Verification items for the finished model (mm, model axes). A direction names the side the tool comes from. Round coordinates to 2 decimals unless told otherwise and drop trailing zeros. Order: outer loops, then holes, each group sorted by start corner. A loop starts at its lowest first (then second) coordinate and runs counter-clockwise, first axis right, second up. Notation, with made-up numbers: (-18.75, 2) -> (35.25, 2) arc R12 cw to (35.25, 23) -> close; hole circle Ø9 at (75.5, 55.5). An arc over 180 degrees is marked (long way). Put each result on its own line as item: value.
```python
from build123d import *

# Parameters (mm, degrees)
BOX_W     = 40
BOX_H     = 40
BOX_DEPTH = 3


with BuildPart() as cono:
    # Cone001 → Cone001 (revolve)
    with BuildSketch(Plane(origin=(0, 0, -4), x_dir=(1, 0, 0), z_dir=(0, -1, 0))):
        Polygon((0, 0), (16, 0), (3, 44), (0, 44), align=None)
    revolve(axis=Axis((0, 0, -4), (0, 0, 1)))


with BuildPart() as cone:
    # Cone → Cone (revolve)
    with BuildSketch(Plane.XZ):
        Polygon((0, 0), (16, 0), (4, 40), (0, 40), align=None)
    revolve(axis=Axis((0, 0, 0), (0, 0, 1)))


with BuildPart() as cut:
    # Box → Box (new body)
    with BuildSketch(Plane(origin=(-20, -20, 0), x_dir=(1, 0, 0), z_dir=(0, 0, 1))):
        with Locations((20, 20)):
            Rectangle(BOX_W, BOX_H)
    extrude(amount=BOX_DEPTH)

    # Fusion: union Cone
    add(cone.part)

    # Cut: cut Cono
    add(cono.part, mode=Mode.SUBTRACT)


solid = cut.part
```
Item 1: Sectioned sample at D-D, the plane y = 16. Record the boundary of the cut face in (x, z).
Geometry check:
outline: (-20, 0) -> (20, 0) -> (20, 3) -> (-20, 3) -> close
Item 2: Depth check by flat-ended pin: pin 1 Ø4 at (x, z) = (-2, 18.5) entering from -Y; pin 2 Ø4 at (y, z) = (10, 28) entering from -X (3 decimals); pin 3 Ø2 at (x, z) = (3, 5) entering from +Y; pin 4 Ø12 at (y, z) = (8, 15) entering from -X. Enter the tip coordinate at first touch or a pass-through.
Geometry check:
pin 1: y = -10.94
pin 2: through
pin 3: y = 14.55
pin 4: x = -12.21
Item 3: Tool access check on faces 4 (the face through (9, 14, 3)), 5 (the face through (-9, 14, 0)). Record the directions out of +Z, -Z, +X, -X, +Y, -Y that give a thin tool (end or side, any length) a straight path to the whole face; none if there is none.
Geometry check:
face 4: +Z
face 5: -Z, +X, -X, +Y, -Y
Item 4: Material ranges on line 1 along Z through (x, y) = (18, 0.5); line 2 along X through (y, z) = (-7, 19); line 3 along Y through (x, z) = (12.5, 4.5), recorded low to high.
Geometry check:
line 1: 0 to 3
line 2: -7.56 to -5.98, 5.98 to 7.56
line 3: -7.64 to -5.07, 5.07 to 7.64
Item 5: Release check for a two-part mould opening along X. For faces 1 (the face through (20, 0, 1)), 2 (the face through (7.166, 2.257, 24.724)), 3 (the face through (0, -20, 1)) record: pulls with the +X half, pulls with the -X half, needs draft (parallel to the pull), parting line crosses it, or undercut.
Geometry check:
face 1: pulls with the +X half
face 2: undercut
face 3: needs draft
Item 6: Sectioned sample at A-A, the plane y = 0. Record the boundary of the cut face in (x, z).
Geometry check:
outline: (-20, 0) -> (-14.82, 0) -> (-3, 40) -> (-4, 40) -> (-15.1, 3) -> (-20, 3) -> close; (3, 40) -> (14.82, 0) -> (20, 0) -> (20, 3) -> (15.1, 3) -> (4, 40) -> close
Item 7: Sectioned sample at C-C, the plane z = 31. Record the boundary of the cut face in (x, y).
Geometry check:
outline: circle Ø13.4 at (0, 0); hole circle Ø11.32 at (0, 0)
